The listing builds one solid part. Answer for the finished solid, in the listing's coordinates (mm). A direction names the side the tool comes from. Coordinates: 2 decimals unless noted, no trailing zeros. Order: outer loops, then holes, each group sorted by start corner. A loop starts at its lowest first (then second) coordinate and runs counter-clockwise, first axis right, second up.
from build123d import *

# Parameters (mm, degrees)
SKETCH1_R           = 0.75
SKETCH1_R_2         = 0.5
BOSS_EXTRUDE1_DEPTH = 4
SKETCH2_W           = 16.2
SKETCH2_H           = 11.795
CUT_EXTRUDE1_DEPTH  = 2


with BuildPart() as part:
    # Sketch1 → Boss-Extrude1 (new body)
    with BuildSketch(Plane.XY):
        with BuildLine():
            Line((0, 6), (0, 11.795))
            ThreePointArc((0, 11.795), (1.464466094, 15.330533906), (5, 16.795))
            Line((5, 16.795), (11.2, 16.795))
            ThreePointArc((11.2, 16.795), (14.735533906, 15.330533906), (16.2, 11.795))
            Line((16.2, 11.795), (16.2, 6))
            Line((16.2, 6), (12.2, 6))
            Line((12.2, 6), (12.2, 4))
            Line((12.2, 4), (16.2, 4))
            Line((16.2, 4), (16.2, 2))
            ThreePointArc((16.2, 2), (15.614213562, 0.585786438), (14.2, 0))
            Line((14.2, 0), (2, 0))
            ThreePointArc((2, 0), (0.585786438, 0.585786438), (0, 2))
            Line((0, 2), (0, 4))
            Line((0, 4), (4, 4))
            Line((4, 4), (4, 6))
            Line((4, 6), (0, 6))
        make_face()
        with Locations(Location((13.45, 2, 0), (0, 0, 180))):
            Circle(SKETCH1_R, mode=Mode.SUBTRACT)
        with Locations((13.45, 8)):
            Circle(SKETCH1_R, mode=Mode.SUBTRACT)
        with Locations((3, 13.795)):
            Circle(SKETCH1_R_2, mode=Mode.SUBTRACT)
        with Locations(Location((13.2, 13.795, 0), (0, 0, 180))):
            Circle(SKETCH1_R_2, mode=Mode.SUBTRACT)
        with Locations(Location((2.75, 8, 0), (0, 0, 180))):
            Circle(SKETCH1_R, mode=Mode.SUBTRACT)
        with Locations((2.75, 2)):
            Circle(SKETCH1_R, mode=Mode.SUBTRACT)
    extrude(amount=BOSS_EXTRUDE1_DEPTH)

    # Sketch2 → Cut-Extrude1 (cut)
    with BuildSketch(Plane.XY):
        with Locations((8.1, 5.8975)):
            Rectangle(SKETCH2_W, SKETCH2_H)
    extrude(amount=CUT_EXTRUDE1_DEPTH, mode=Mode.SUBTRACT)


solid = part.part
(1) A tool of negligible diameter and unlimited length cuts with its end or side. For faces 5 (the flat face through (14, 4, 3)), 6 (the flat face through (2, 6, 3)), 7 (the flat face through (8, 11.795, 1)), from which of +Z, -Z, +X, -X, +Y, -Y can it reach the whole face along a straight path? Write none if from no direction.
(2) Find the intervals of material crossed by probe 1 along X at (y, z) = (8, 3.5); probe 2 along Y at (x, z) = (2.75, 2.8); probe 3 along Y at (x, z) = (13.2, 2.9) (3 decimals), in increasing order.
(3) Find section B-B on x = 13.45. Determine the outline of the cut face in (y, z) (3 decimals).
(4) The mould has two halves that part along Y. Classify faces 1 (the cylindrical face through (2.2, 2.51, 2.99)), 2 (the cylindrical face through (14.165, 8.225, 2.986)), 3 (the flat face through (8, 14, 0)), 4 (the flat face through (8, 16.795, 2)): pulls with the +Y half, pulls with the -Y half, needs draft (parallel to the pull), parting line crosses it, or undercut.
(5) Given pin 1 Ø2 at (x, z) = (15, 3) entering from +Y; pin 2 Ø1 at (x, z) = (1.5, 3) entering from +Y (3 decimals); pin 3 Ø9.5 at (x, y) = (4, 5) entering from -Z, each flat-ended and moving along its own axis, determine where each tip first touches the part or whether it passes through.
(6) Find section C-C on z = 2.3. Determine the outline of the cut face in (x, y) (3 decimals), then the cut area to 3 significant figures.
(7) Find section D-D on z = 0.3. Determine the outline of the cut face in (x, y) (3 decimals).
(8) Find section A-A on y = 8. Determine the outline of the cut face in (x, z), then the cut area to 3 significant figures.
Resolved:
1. face 5: +Z, -Z, +X
1. face 6: +Z, -Z, -X
1. face 7: -Z, +X, -X, -Y
2. probe 1: x = 0 to 2, 3.5 to 12.7, 14.2 to 16.2
2. probe 2: y = 0 to 1.25, 2.75 to 4, 6 to 7.25, 8.75 to 13.36, 14.23 to 16.26
2. probe 3: y = 0 to 1.293, 2.707 to 4, 6 to 7.293, 8.707 to 13.295, 14.295 to 16.378
3. outline: (0, 2) - (1.25, 2) - (1.25, 4) - (0, 4) - close; (2.75, 2) - (4, 2) - (4, 4) - (2.75, 4) - close; (6, 2) - (7.25, 2) - (7.25, 4) - (6, 4) - close; (8.75, 2) - (11.795, 2) - (11.795, 0) - (13.362, 0) - (13.362, 4) - (8.75, 4) - close; (14.228, 0) - (16.26, 0) - (16.26, 4) - (14.228, 4) - close
4. face 1: undercut
4. face 2: undercut
4. face 3: needs draft
4. face 4: pulls with the +Y half
5. pin 1: stops at y = 15.94
5. pin 2: stops at y = 15.795
5. pin 3: stops at z = 2
6. outline: (0, 2) arc R2 ccw to (2, 0) - (14.2, 0) arc R2 ccw to (16.2, 2) - (16.2, 4) - (12.2, 4) - (12.2, 6) - (16.2, 6) - (16.2, 11.795) arc R5 ccw to (11.2, 16.795) - (5, 16.795) arc R5 ccw to (0, 11.795) - (0, 6) - (4, 6) - (4, 4) - (0, 4) - close; hole circle Ø1.5 at (2.75, 2); hole circle Ø1.5 at (2.75, 8); hole circle Ø1 at (3, 13.795); hole circle Ø1.5 at (13.45, 2); hole circle Ø1.5 at (13.45, 8); hole circle Ø1 at (13.2, 13.795)
6. area: 235 mm2
7. outline: (0, 11.795) - (16.2, 11.795) arc R5 ccw to (11.2, 16.795) - (5, 16.795) arc R5 ccw to start; hole circle Ø1 at (3, 13.795); hole circle Ø1 at (13.2, 13.795)
8. outline: (0, 2) - (2, 2) - (2, 4) - (0, 4) - close; (3.5, 2) - (12.7, 2) - (12.7, 4) - (3.5, 4) - close; (14.2, 2) - (16.2, 2) - (16.2, 4) - (14.2, 4) - close
8. area: 26.4 mm2
